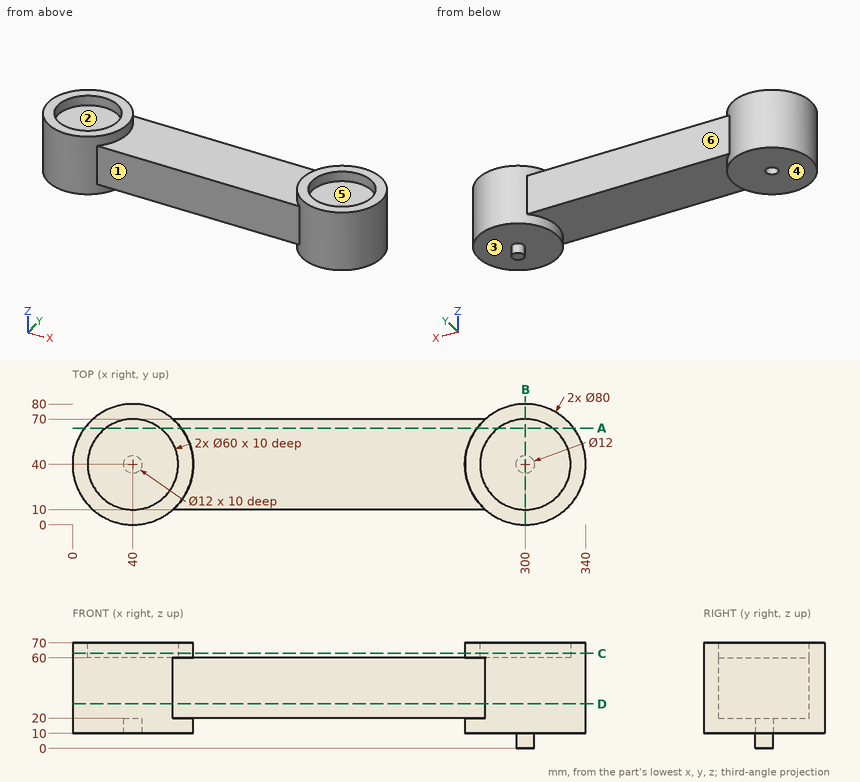
Check sheet for the drawn part. Datum: minimum x, y, z corner. Units: mm. A direction names the side the tool comes from. Round coordinates to 2 decimals unless told otherwise and drop trailing zeros. Order: outer loops, then holes, each group sorted by start corner. A loop starts at its lowest first (then second) coordinate and runs counter-clockwise, first axis right, second up. Notation, with made-up numbers: (86, 80) -> (101, 80) arc R27 cw to (101, 119) -> close; hole circle Ø4 at (41, 36.25). An arc over 180 degrees is marked (long way). Return JSON: item names as keys, results as strings. Group by question number.
Q1. Release check for a two-part mould opening along Y. For the marked faces 1, 2 and 3 record: released by +Y, released by -Y, zero draft, split by the parting line, or undercut.
Q2. Section check B-B, the plane x = 300. Record the boundary of the cut face in (y, z), plus the area to 3 significant figures.
Q3. Gauge pin test, flat ends, axial feed: pin 1 (1.5 mm diameter, centred on y = 21, z = 47.5, fed in from -X); pin 2 (6 mm diameter, centred on y = 16, z = 12, fed in from -X); pin 3 (12 mm diameter, centred on x = 199.5, z = 42, fed in from -Y). Record the tip position at first contact, or that the pin passes through.
Q4. Material ranges on probe 1 along Y at (x, z) = (40, 16); probe 2 along Y at (x, z) = (300, 63.75); probe 3 along Z at (x, y) = (291.5, 62), recorded low to high. Write a range as from..to.
Q5. Tool access check on the marked faces 4, 5 and 6. Record the directions out of +Z, -Z, +X, -X, +Y, -Y that give a thin tool (end or side, any length) a straight path to the whole face; none if there is none.
Q6. Section check D-D, the plane z = 29.5. Record the boundary of the cut face in (x, y), plus the area to 3 significant figures.
Q7. Section check A-A, the plane y = 64. Record the boundary of the cut face in (x, z).
Q8. Section check C-C, the plane z = 63. Record the boundary of the cut face in (x, y).
Numbers:
{
 "1": {"face 1": "released by -Y", "face 2": "undercut", "face 3": "zero draft"},
 "2": {"outline": "(0, 10) -> (34, 10) -> (34, 0) -> (46, 0) -> (46, 10) -> (80, 10) -> (80, 70) -> (70, 70) -> (70, 60) -> (10, 60) -> (10, 70) -> (0, 70) -> close", "area": "4,320 mm^2"},
 "3": {"pin 1": "x = 4.41", "pin 2": "x = 5.96", "pin 3": "y = 10"},
 "4": {"probe 1": "0..34, 46..80", "probe 2": "0..10, 70..80", "probe 3": "10..60"},
 "5": {"face 4": "-Z, -X, +Y, -Y", "face 5": "+Z", "face 6": "+Z, -Z, +Y"},
 "6": {"outline": "(66.46, 10) -> (273.54, 10) arc R40 ccw (long way) to (273.54, 70) -> (66.46, 70) arc R40 ccw (long way) to start", "area": "21,400 mm^2"},
 "7": {"outline": "(8, 10) -> (72, 10) -> (72, 20) -> (268, 20) -> (268, 10) -> (332, 10) -> (332, 70) -> (318, 70) -> (318, 60) -> (282, 60) -> (282, 70) -> (268, 70) -> (268, 60) -> (72, 60) -> (72, 70) -> (58, 70) -> (58, 60) -> (22, 60) -> (22, 70) -> (8, 70) -> close"},
 "8": {"outline": "circle Ø80 at (40, 40); circle Ø80 at (300, 40); hole circle Ø60 at (40, 40); hole circle Ø60 at (300, 40)"}
}
